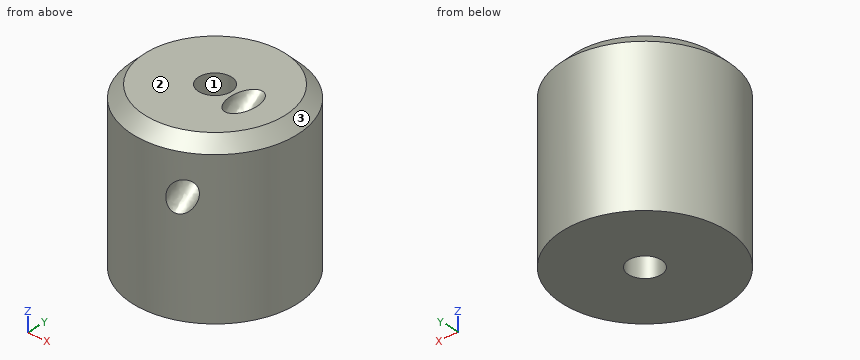
```python
from build123d import *

# Parameters (mm, degrees)
F0_R     = 10
F0_R_2   = 2
F1_DEPTH = 20
F5_R     = 1.5
F7_SIZE  = 1.5


with BuildPart() as f1:
    # F0 (on Top) → F1 (new body)
    with BuildSketch(Plane.XY):
        Circle(F0_R)
        Circle(F0_R_2, mode=Mode.SUBTRACT)
    extrude(amount=F1_DEPTH)

    # F6: sweep along a path in F3
    with BuildLine(Plane.YZ.offset(4)) as f6_path:
        Line((3.480567, 22.941271), (-17.466422, 7.439554))
    # F5 (on face) → F6 (sweep, cut)
    with BuildSketch(Plane(origin=(0, 13.2187, 9.782434), x_dir=(1, 0, 0), z_dir=(0, -0.803825, -0.594866))):
        with Locations((4, 16.370284)):
            Circle(F5_R)
    sweep(path=f6_path.line, mode=Mode.SUBTRACT)

    # F7
    f7_edges = [f1.edges().sort_by_distance(p)[0] for p in [
        (-10, 0, 20),
    ]]
    chamfer(f7_edges, length=F7_SIZE)


solid = f1.part
```
Here's how the part is built. I have some questions about the finished solid (model axes, mm). Face numbers are marked on the shaded views. Give positions to 0.01 mm unless a question says otherwise; leave off trailing zeros. Order: outer loops, then holes, each group sorted by start corner. A loop starts at its lowest first (then second) coordinate and runs counter-clockwise, first axis right, second up. Notation, with made-up numbers: (33, 68) - (78, 68) arc R19 ccw to (78, 78) - close; hole circle Ø2 at (66.25, 37.25). An arc over 180 degrees is marked (long way). Answer as a JSON object with one key per item and string values. Group by question number.
Item 1: If we section it at A-A on x = 0: Please give me the cut outline in (y, z).
Item 2: Please list where these lines run through material, in increasing order: probe 1 along Y at (x, z) = (0, 15.5); probe 2 along Y at (x, z) = (-1.25, 15.25); probe 3 along X at (y, z) = (-1, 5.25).
Item 3: If we mould it in two halves opening along X, with no side actions, what happens to the marked faces 1, 2 and 3? For each: pulls with the +X half, pulls with the -X half, needs draft (parallel to the pull), parting line crosses it, or undercut.
Item 4: If we section it at B-B on z = 11.25: Please give me the cut outline in (x, y), and give its area (3 significant figures).
Item 5: For P1, Ø1, axis at x = 3.5, y = -1.5, coming from the +Z side; P2, Ø2, axis at x = 4, z = 15.5, coming from the -Y side; P3, Ø1.5, axis at x = 4.5, z = 10, coming from the -Y side, each with a flat end and sliding along its axis, tell me the tip position at first contact or that it passes through.
Result set:
{
 "1": {"outline": "(-10, 0) - (-2, 0) - (-2, 20) - (-8.5, 20) - (-10, 18.5) - close; (2, 0) - (10, 0) - (10, 18.5) - (8.5, 20) - (2, 20) - close"},
 "2": {"probe 1": "-10 to -2, 2 to 10", "probe 2": "-9.92 to -1.56, 1.56 to 9.92", "probe 3": "-9.95 to -1.73, 1.73 to 9.95"},
 "3": {"face 1": "undercut", "face 2": "needs draft", "face 3": "parting line crosses it"},
 "4": {"outline": "circle Ø20 at (0, 0); hole circle Ø4 at (0, 0)", "area": "302 mm²"},
 "5": {"P1": "z = 17.98", "P2": "y = -9.54", "P3": "y = -9.27"}
}
